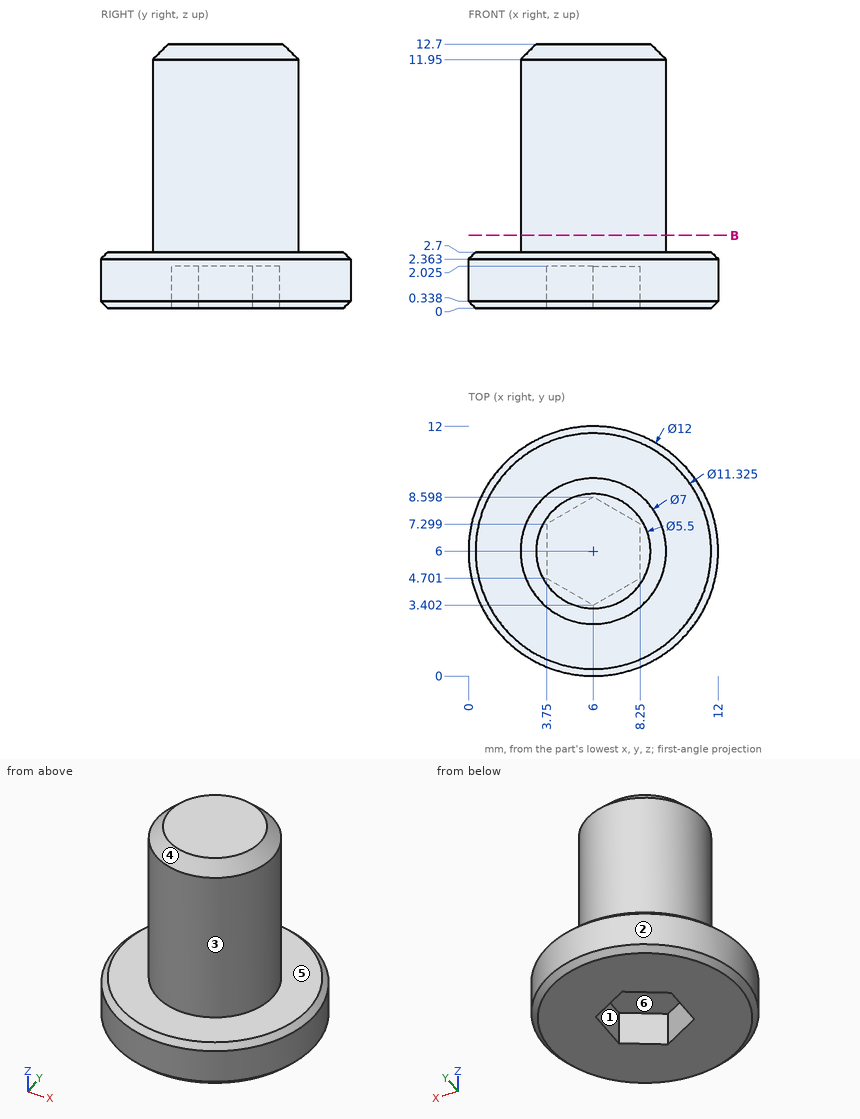
Drawing for the job (mm, zero at the part's lowest x, y, z). A direction names the side the tool comes from. Round coordinates to 2 decimals unless told otherwise and drop trailing zeros. Write each loop counter-clockwise with the first axis right and the second up, starting at its lowest first coordinate (ties: lowest second). Pieces come first, ordered by that corner, then holes. Notation, with made-up numbers: (32.5, 27) - (75.5, 27) arc R23 ccw to (75.5, 44) - close; hole circle Ø3 at (75.5, 43.25). An arc over 180 degrees is marked (long way). Write item = value, one per line. Start each with the question number.
Q1. Probe L1, parallel to Z at x = 5.25, y = 10.25; L2, parallel to Z at x = 6.75, y = 4 (1 decimal); L3, parallel to Y at x = 1.25, z = 0.75 (1 decimal). List the from-to ranges inside material, lowest first. Write a range as from..to.
Q2. Drop flat-ended pins along their axis: pin 1 (5 mm diameter, centred on x = 9.5, z = 6, fed in from +Y) (1 decimal); pin 2 (1.5 mm diameter, centred on y = 3.5, z = 7, fed in from -X); pin 3 (2 mm diameter, centred on x = 4.5, z = 8.5, fed in from -Y). Give the stop position or say it passes through.
Q3. Mould opens along X. For the marked faces 4, 5 and 6 say: pulls with the +X half, pulls with the -X half, needs draft (parallel to the pull), parting line crosses it, or undercut.
Q4. Which spindle directions (+Z, -Z, +X, -X, +Y, -Y) get a long thin tool onto all of the face, cutting with end or side? Do the marked faces 1, 2 and 3. Say none if no direction does.
Q5. Band-saw the part on B-B (z = 3.5). Give the cut face in (x, y), then the cut area to 3 significant figures.
Answers below:
q1.L1 = 0..2.7
q1.L2 = 2..12.7
q1.L3 = 2.3..9.7
q2.pin_1 = 9.4
q2.pin_2 = 2.97
q2.pin_3 = 2.54
q3.face_4 = parting line crosses it
q3.face_5 = needs draft
q3.face_6 = undercut
q4.face_1 = -Z
q4.face_2 = +Z, -Z
q4.face_3 = +Z
q5.outline = circle Ø7 at (6, 6)
q5.area = 38.5 mm2
